from build123d import *

# Parameters (mm, degrees)
SKETCH_1_R               = 15
EXTRUDE_1_DEPTH          = 5
CUT_EXTRUDE_1_DEPTH      = 30
CUT_EXTRUDE_2_DEPTH      = 60
SKETCH_4_R               = 1
EXTRUDE_2_DEPTH          = 5
SKETCH_5_W               = 3
SKETCH_5_H               = 5.040496026
CUT_EXTRUDE_3_DEPTH      = 28.39432933
CUT_EXTRUDE_4_DEPTH      = 28.39432933
CUT_EXTRUDE_4_DEPTH_BACK = 28.39432933
SKETCH_6_W               = 3
SKETCH_6_H               = 1.5


with BuildPart() as part:
    # 草图1 → 凸台-拉伸1 (new body)
    with BuildSketch(Plane.XY):
        Circle(SKETCH_1_R)
    extrude(amount=EXTRUDE_1_DEPTH)

    # 草图2 → 切除-拉伸1 (cut)
    with BuildSketch(Plane.XY.offset(5)):
        Polygon((-2.5, -4.330127019), (2.5, -4.330127019), (5, 0), (2.5, 4.330127019), (-2.5, 4.330127019), (-5, 0), align=None)
    extrude(amount=-CUT_EXTRUDE_1_DEPTH, mode=Mode.SUBTRACT)

    # 草图3 → 切除-拉伸2 (cut)
    with BuildSketch(Plane.XY.offset(5)):
        Polygon((-8.586571111, 14), (9.123789919, 14), (-0.951474436, 18.675160858), align=None)
    extrude(amount=-CUT_EXTRUDE_2_DEPTH, mode=Mode.SUBTRACT)

    # 草图4 → 凸台-拉伸2 (add)
    with BuildSketch(Plane.XY.offset(5)):
        with BuildLine():
            Line((5.385164807, 14), (5.26595559, 15.333555474))
            ThreePointArc((5.26595559, 15.333555474), (4.293622117, 16.606349783), (2.726438877, 16.275631735))
            Line((2.726438877, 16.275631735), (0.385164807, 14))
            Line((0.385164807, 14), (5.385164807, 14))
        make_face()
        with Locations((3.771913109, 15.2)):
            Circle(SKETCH_4_R, mode=Mode.SUBTRACT)
    extrude(amount=-EXTRUDE_2_DEPTH)

    # 草图5 → 切除-拉伸3 (cut, through all)
    with BuildSketch(Plane(origin=(6.584040452, 0.588560672, 0), x_dir=(0, 0, -1), z_dir=(0.996028320712149, 0.08903698298648982, 0))):
        with Locations((-2.5, 15.985165676)):
            Rectangle(SKETCH_5_W, SKETCH_5_H)
    extrude(amount=-CUT_EXTRUDE_3_DEPTH, mode=Mode.SUBTRACT)

    # 草图6 → 切除-拉伸4 (cut, two sides: drawn at the far end of the back side and taken through both)
    with BuildSketch(Plane(origin=(6.584040452, 0.588560672, 0), x_dir=(0, 0, -1), z_dir=(0.996028320712149, 0.08903698298649015, 0)).offset(-CUT_EXTRUDE_4_DEPTH_BACK)):
        with Locations((-2.5, 12.714917663)):
            Rectangle(SKETCH_6_W, SKETCH_6_H)
    extrude(amount=CUT_EXTRUDE_4_DEPTH + CUT_EXTRUDE_4_DEPTH_BACK, mode=Mode.SUBTRACT)


solid = part.part
Geometry: final body of the model. Coordinates: model frame, mm. A direction names the side the tool comes from. Give positions to 0.01 mm unless a question says otherwise; leave off trailing zeros. Write each loop counter-clockwise with the first axis right and the second up, starting at its lowest first coordinate (ties: lowest second). Pieces come first, ordered by that corner, then holes. Notation, with made-up numbers: (-38, 28.5) - (17, 28.5) arc R27 ccw to (17, 61.5) - close; hole circle Ø3 at (-2, 24.25). An arc over 180 degrees is marked (long way). Return JSON: item names as keys, results as strings. Group by question number.
1) Section B-B on x = 0. Return the cut outline in (y, z).
2) Section A-A on z = 2.65. Return the cut outline in (x, y), plus the area to 3 significant figures.
3) Section C-C on y = 0.5. Return the cut outline in (x, z).
4) First-contact query: P1, Ø2, axis at y = 7, z = 4, coming from the -X side; P2, Ø2.5, axis at x = 0.5, z = 3.5, coming from the +Y side; P3, Ø1.1, axis at x = -3.5, z = 0.5, coming from the +Y side; P4, Ø3, axis at x = -0.5, y = -2, coming from the -Z side. Flat tips, straight axial feed; report the tip coordinate or a pass-through.
5) Line query: line 1 (Y direction, x = -0.25, z = 4.1); line 2 (Z direction, x = -5, y = 12.5); line 3 (Y direction, x = 2.25, z = 0.9). Output: solid intervals per line, ascending.
6) Section D-D on x = -8.5. Return the cut outline in (y, z).
7) Set-up query: faces 4 (the flat face through (0, -4.33, 3)), 5 (the flat face through (-1.191, 11.906, 2.521)), 6 (the flat face through (5.326, 14.657, 0.507)). Return all of +Z, -Z, +X, -X, +Y, -Y with unobstructed straight access to the full face (end or side cutting, diameter ignored); none if empty.
8) Mould query, pull axis Y, two halves, no side actions, for faces 1 (the flat face through (0, 5, 0)), 2 (the cylindrical face through (-0.58, -14.99, 2.46)), 3 (the cylindrical face through (3.555, 14.224, 0.507)). Classes: released by +Y, released by -Y, zero draft, split by the parting line, or undercut.
Filled in:
{
 "1": {"outline": "(-15, 0) - (-4.33, 0) - (-4.33, 5) - (-15, 5) - close; (4.33, 0) - (14, 0) - (14, 1) - (12.01, 1) - (12.01, 4) - (14, 4) - (14, 5) - (4.33, 5) - close"},
 "2": {"outline": "(-10.08, 11.11) arc R15 ccw (long way) to (7.95, 12.72) - close; hole (-5, 0) - (-2.5, -4.33) - (2.5, -4.33) - (5, 0) - (2.5, 4.33) - (-2.5, 4.33) - close", "area": "604 mm^2"},
 "3": {"outline": "(-14.99, 0) - (-4.71, 0) - (-4.71, 5) - (-14.99, 5) - close; (4.71, 0) - (14.99, 0) - (14.99, 5) - (4.71, 5) - close"},
 "4": {"P1": "stops at x = -13.75", "P2": "stops at y = 15.23", "P3": "stops at y = 14", "P4": "passes through"},
 "5": {"line 1": "y = -15 to -4.33, 4.33 to 14", "line 2": "z = 0 to 1, 4 to 5", "line 3": "y = -14.83 to -4.33, 4.33 to 15.81"},
 "6": {"outline": "(-12.36, 0) - (12.36, 0) - (12.36, 1) - (11.25, 1) - (11.25, 4) - (12.36, 4) - (12.36, 5) - (-12.36, 5) - close"},
 "7": {"face 4": "+Z, -Z", "face 5": "-X, +Y", "face 6": "+Z, -Z, +X, +Y"},
 "8": {"face 1": "zero draft", "face 2": "split by the parting line", "face 3": "undercut"}
}
